The figure shows three views and two pictorial views of one solid part (mm, origin at its lowest corner). Answer the questions. Give positions to 0.01 mm unless a question says otherwise; leave off trailing zeros. Write each loop counter-clockwise with the first axis right and the second up, starting at its lowest first coordinate (ties: lowest second). Pieces come first, ordered by that corner, then holes. Notation, with made-up numbers: (51.5, -9) - (109.5, -9) arc R24 ccw to (109.5, 13) - close; hole circle Ø3 at (28, 76.5). An arc over 180 degrees is marked (long way). One line per question, with ' | ' between items. Start each with the question number.
1. The mould has two halves that part along X. Classify the marked faces 1, 2, 3 and 4: +X half, -X half, draft (parallel to the pull), parting line (faces both ways), or undercut.
2. A cutting plane is placed at B-B (y = 47.3). Determine the outline of the cut face in (x, z).
3. A cutting plane is placed at A-A (x = 24). Determine the outline of the cut face in (y, z).
4. Given P1, Ø4.5, axis at x = 12, z = 10, coming from the +Y side; P2, Ø4.5, axis at x = 37.44, z = 10.06, coming from the +Y side, each flat-ended and moving along its own axis, determine where each tip first touches the part or whether it passes through.
5. A cutting plane is placed at D-D (z = 23.5). Determine the outline of the cut face in (x, y), then the cut area to 3 significant figures.
6. A cutting plane is placed at C-C (z = 42.5). Determine the outline of the cut face in (x, y), then the cut area to 3 significant figures.
7. Find the intervals of material crossed by L1, parallel to Z at x = 24, y = 60; L2, parallel to Y at x = 45.5, z = 40.5; L3, parallel to Z at x = 19, y = 46, in increasing order. Write a range as from..to.
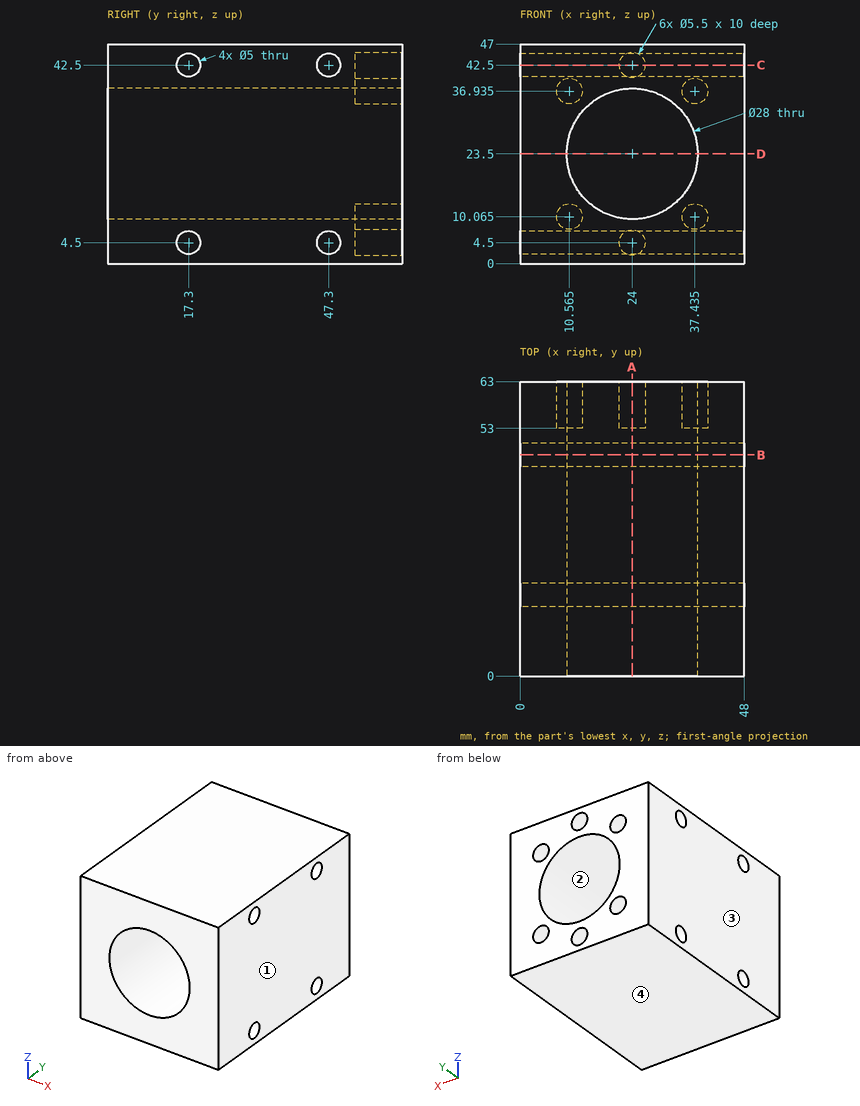
Determined:
1) face 1: +X half | face 2: undercut | face 3: -X half | face 4: draft
2) outline: (0, 0) - (48, 0) - (48, 2) - (0, 2) - close; (0, 7) - (48, 7) - (48, 40) - (0, 40) - close; (0, 45) - (48, 45) - (48, 47) - (0, 47) - close; hole circle Ø28 at (24, 23.5)
3) outline: (0, 0) - (63, 0) - (63, 1.75) - (53, 1.75) - (53, 7.25) - (63, 7.25) - (63, 9.5) - (0, 9.5) - close; (0, 37.5) - (63, 37.5) - (63, 39.75) - (53, 39.75) - (53, 45.25) - (63, 45.25) - (63, 47) - (0, 47) - close; hole circle Ø5 at (17.3, 4.5); hole circle Ø5 at (17.3, 42.5); hole circle Ø5 at (47.3, 4.5); hole circle Ø5 at (47.3, 42.5)
4) P1: y = 63 | P2: y = 53
5) outline: (0, 0) - (10, 0) - (10, 63) - (0, 63) - close; (38, 0) - (48, 0) - (48, 63) - (38, 63) - close | area: 1,260 mm2
6) outline: (0, 0) - (48, 0) - (48, 14.8) - (0, 14.8) - close; (0, 19.8) - (48, 19.8) - (48, 44.8) - (0, 44.8) - close; (0, 49.8) - (48, 49.8) - (48, 63) - (26.75, 63) - (26.75, 53) - (21.25, 53) - (21.25, 63) - (0, 63) - close | area: 2,490 mm2
7) L1: 0..1.75, 7.25..9.5, 37.5..39.75, 45.25..47 | L2: 0..15.8, 18.8..45.8, 48.8..63 | L3: 0..2.36, 6.64..10.42, 36.58..40.36, 44.64..47
